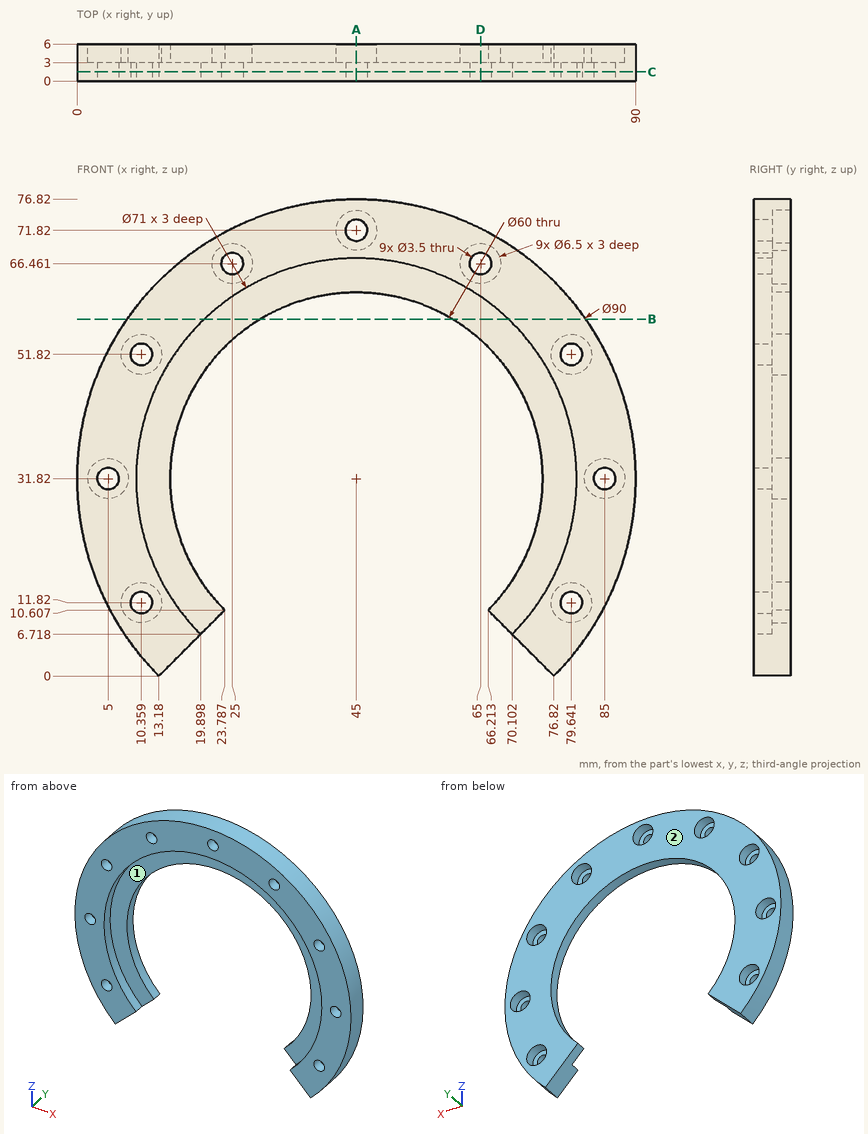
Could you check a few things on this drawing? It's one solid part, dimensions in mm from its lowest x, y, z. A direction names the side the tool comes from. Coordinates: 2 decimals unless noted, no trailing zeros. Order: outer loops, then holes, each group sorted by start corner. A loop starts at its lowest first (then second) coordinate and runs counter-clockwise, first axis right, second up.
1. For the marked faces 1 and 2, which set-ups out of +Z, -Z, +X, -X, +Y, -Y let a thin tool reach every point of the face, with its end or its side?
2. If we section it at C-C (y = 1.5): Give the number of separate pieces and of enclosed holes in the cut face.
3. If we section it at A-A (x = 45): Please give me the cut outline in (y, z).
4. I need wall thicknesses on line 1 (X direction, y = 5, z = 14.5) (1 decimal); line 2 (Y direction, x = 23.5, z = 57); line 3 (Z direction, x = 45, y = 2.1). Which ranges of each line are inside material? Lowest first, please.
5. If we section it at D-D (x = 65): Please give me the cut outline in (y, z).
6. If we section it at B-B (z = 57.5): Please give me the cut outline in (x, y).
7. I'm going to push flat-ended pins straight in: pin 1 (3 mm diameter, centred on x = 65, z = 66.46, fed in from -Y); pin 2 (1.5 mm diameter, centred on x = 57.5, z = 62, fed in from -Y); pin 3 (2 mm diameter, centred on x = 66, z = 65, fed in from +Y). Where does each tip first touch, or does it pass through?
Entries:
1. face 1: -Y
1. face 2: +Z, -Z, +X, -X, +Y
2. separate pieces: 1
2. enclosed holes: 9
3. outline: (0, 67.32) - (3, 67.32) - (3, 61.82) - (6, 61.82) - (6, 68.57) - (3, 68.57) - (3, 70.07) - (0, 70.07) - close; (0, 73.57) - (3, 73.57) - (3, 75.07) - (6, 75.07) - (6, 76.82) - (0, 76.82) - close
4. line 1: x = 3.5 to 8.5, 12.2 to 20.5, 69.5 to 77.8, 81.5 to 86.5
4. line 2: y = 3 to 6
4. line 3: z = 67.32 to 70.07, 73.57 to 76.82
5. outline: (0, 61.15) - (3, 61.15) - (3, 54.18) - (6, 54.18) - (6, 63.21) - (3, 63.21) - (3, 64.71) - (0, 64.71) - close; (0, 68.21) - (3, 68.21) - (3, 69.71) - (6, 69.71) - (6, 72.13) - (0, 72.13) - close
6. outline: (8.05, 0) - (20.49, 0) - (20.49, 3) - (29.49, 3) - (29.49, 6) - (8.05, 6) - close; (60.51, 3) - (69.51, 3) - (69.51, 0) - (81.95, 0) - (81.95, 6) - (60.51, 6) - close
7. pin 1: passes through
7. pin 2: stops at y = 3
7. pin 3: stops at y = 3
